Model file for the job. Use its own axes, mm. Face numbers are marked on the shaded views. A direction names the side the tool comes from. Give positions to 0.01 mm unless a question says otherwise; leave off trailing zeros. Order: outer loops, then holes, each group sorted by start corner. A loop starts at its lowest first (then second) coordinate and runs counter-clockwise, first axis right, second up. Notation, with made-up numbers: (77.25, 16) -> (136.25, 16) arc R30 ccw to (136.25, 53) -> close; hole circle Ø8 at (40.5, 34). An arc over 180 degrees is marked (long way). Use CSV: the item, a comma, the result in double quotes. Start each with the question number.
1. 3-axis set-ups, long thin cutter, end or side, ignore diameter. For the marked faces 1 and 2: which of +Z, -Z, +X, -X, +Y, -Y reach the whole face in a straight line?
2. Drop flat-ended pins along their axis: pin 1 (1.1 mm diameter, centred on y = 14.5, z = -11.5, fed in from -X); pin 2 (0.8 mm diameter, centred on y = 14.5, z = -10, fed in from +X); pin 3 (5.5 mm diameter, centred on x = 0, z = -10.5, fed in from -Y); pin 4 (4 mm diameter, centred on x = 3, z = -1.5, fed in from -Y). Give the stop position or say it passes through.
3. Cut at A-A on x = 0. List the corners of the cut face in (y, z), then the cut area to 3 significant figures.
4. Wall check: line 1 (Z direction, x = 0, y = 14.55); line 2 (Z direction, x = -4.75, y = 5.5); line 3 (X direction, y = 14.5, z = -2.75). Give the ranges that are in metal, low to high. Write a range as from..to.
5. Cut at B-B on z = -18.5. List the corners of the cut face in (x, y).
6. Cut at D-D on y = 8. List the corners of the cut face in (x, z), then the cut area to 3 significant figures.
7. Cut at C-C on x = 8. List the corners of the cut face in (y, z).
```python
from build123d import *

# Parameters (mm, degrees)
SKETCH1_W           = 23
SKETCH1_H           = 5
BOSS_EXTRUDE1_DEPTH = 15
SKETCH3_R           = 1
BOSS_EXTRUDE4_DEPTH = 1


with BuildPart() as part:
    # Sketch1 → Boss-Extrude1 (new body)
    with BuildSketch(Plane(origin=(0, 0, 0), x_dir=(1, 0, 0), z_dir=(0, 1, 0))):
        Rectangle(SKETCH1_W, SKETCH1_H)
    extrude(amount=BOSS_EXTRUDE1_DEPTH)

    # Sketch3 → Boss-Extrude4 (add)
    with BuildSketch(Plane(origin=(0, 15, 0), x_dir=(1, 0, 0), z_dir=(0, 1, 0))):
        with BuildLine():
            Line((-3.5, 19.5), (-3.5, 2.5))
            Line((-3.5, 2.5), (3.5, 2.5))
            Line((3.5, 2.5), (3.5, 19.5))
            ThreePointArc((3.5, 19.5), (0, 22.488926095), (-3.5, 19.5))
        make_face()
        with Locations((0, 18.945232051)):
            Circle(SKETCH3_R, mode=Mode.SUBTRACT)
    extrude(amount=-BOSS_EXTRUDE4_DEPTH)


solid = part.part
```
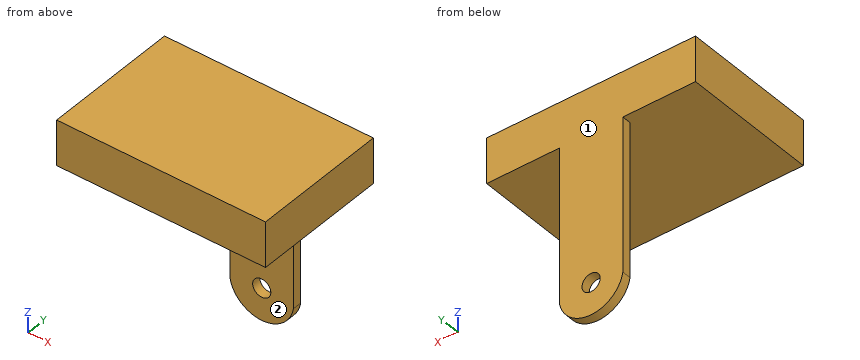
Verdict:
1,face 1,"+Z, -Z, +X, -X, +Y"
1,face 2,"-Z, +X, -X, -Y"
2,pin 1,"x = -3.5"
2,pin 2,"x = 3.5"
2,pin 3,"y = 14"
2,pin 4,"y = 0"
3,outline,"(0, -2.5) -> (14, -2.5) -> (14, -17.95) -> (15, -17.95) -> (15, 2.5) -> (0, 2.5) -> close; (14, -22.49) -> (15, -22.49) -> (15, -19.95) -> (14, -19.95) -> close"
3,area,"93.0 mm^2"
4,line 1,"-22.49..-19.95, -17.95..2.5"
4,line 2,"-2.5..2.5"
4,line 3,"-3.5..3.5"
5,outline,"(-3.5, 14) -> (-0.9, 14) -> (-0.9, 15) -> (-3.5, 15) -> close; (0.9, 14) -> (3.5, 14) -> (3.5, 15) -> (0.9, 15) -> close"
6,outline,"(-11.5, -2.5) -> (11.5, -2.5) -> (11.5, 2.5) -> (-11.5, 2.5) -> close"
6,area,"115 mm^2"
7,outline,"(0, -2.5) -> (15, -2.5) -> (15, 2.5) -> (0, 2.5) -> close"
